Work out the finished part from the listing and answer in its coordinate system (mm). A direction names the side the tool comes from. Coordinates: 2 decimals unless noted, no trailing zeros. Loops run counter-clockwise (first coordinate to the right, second up) from the corner with the lowest first, then second, coordinate; pieces in that order, holes last. Notation, with made-up numbers: (13.25, 4) - (17.25, 4) arc R19 ccw to (17.25, 11) - close; hole circle Ø8 at (21.25, 62). An arc over 180 degrees is marked (long way). Write each question's results on one line, items separated by ' | '. Start each with the question number.
1. A cutting plane is placed at A-A on y = -6.25. Determine the outline of the cut face in (x, z).
2. Determine the mould class of faces 1 (the cylindrical face through (8.69, -5.26, 1.48)), 2 (the cylindrical face through (-6.31, -5.26, 1.48)), 3 (the flat face through (0, 9, 9)), 4 (the flat face through (-15.5, 0, 9)) for opening direction Y: released by +Y, released by -Y, zero draft, split by the parting line, or undercut.
3. Which of the six approach directions +Z, -Z, +X, -X, +Y, -Y give full straight-line access (tool end or side, diameter ignored) to faces 5 (the flat face through (15.5, 0, 9)), 6 (the flat face through (0, 2, 4.4)), 7 (the flat face through (0, 0, 12))?
4. A cutting plane is placed at D-D on z = 16.5. Determine the outline of the cut face in (x, y).
5. A cutting plane is placed at B-B on x = 7.5. Determine the outline of the cut face in (y, z).
6. Each of these flat-tipped pins is pushed along its axis until it touches: P1, Ø4.5, axis at x = -7, y = -5, coming from the +Z side; P2, Ø6, axis at x = -6, z = 14, coming from the -Y side. Where does it stop, or does it pass through?
7. A cutting plane is placed at C-C on y = 0.5. Determine the outline of the cut face in (x, z), then the cut area to 3 significant figures.
8. Find the intervals of material crossed by line 1 along X through (y, z) = (-4.25, 4.75); line 2 along Y through (x, z) = (7.5, 1.55); line 3 along Z through (x, y) = (2.5, 3), in increasing order. Write a range as [from, to].
from build123d import *

# Parameters (mm, degrees)
CROQUIS1_W              = 31
CROQUIS1_H              = 18
SALIENTE_EXTRUIR1_DEPTH = 19
CROQUIS3_W              = 25.1
CROQUIS3_H              = 9
CORTAR_EXTRUIR1_DEPTH   = 16
CROQUIS4_W              = 31
CROQUIS4_H              = 1.4
CORTAR_EXTRUIR2_DEPTH   = 15.1
CROQUIS5_R              = 1.5
CORTAR_EXTRUIR3_DEPTH   = 20


with BuildPart() as part:
    # Croquis1 → Saliente-Extruir1 (new body)
    with BuildSketch(Plane.XY):
        Rectangle(CROQUIS1_W, CROQUIS1_H)
    extrude(amount=SALIENTE_EXTRUIR1_DEPTH)

    # Croquis3 → Cortar-Extruir1 (cut)
    with BuildSketch(Plane.XY.offset(19)):
        with Locations((0, -4.5)):
            Rectangle(CROQUIS3_W, CROQUIS3_H)
    extrude(amount=-CORTAR_EXTRUIR1_DEPTH, mode=Mode.SUBTRACT)

    # Croquis4 → Cortar-Extruir2 (cut)
    with BuildSketch(Plane.XZ.offset(9)):
        with Locations((0, 3.7)):
            Rectangle(CROQUIS4_W, CROQUIS4_H)
    extrude(amount=-CORTAR_EXTRUIR2_DEPTH, mode=Mode.SUBTRACT)

    # Croquis5 → Cortar-Extruir3 (cut, through all)
    with BuildSketch(Plane(origin=(0, 0, 0), x_dir=(-1, 0, 0), z_dir=(0, 0, -1))):
        with Locations((-7.5, -4.35)):
            Circle(CROQUIS5_R)
        with Locations((7.5, -4.35)):
            Circle(CROQUIS5_R)
    extrude(amount=-CORTAR_EXTRUIR3_DEPTH, mode=Mode.SUBTRACT)


solid = part.part
Values:
1) outline: (-15.5, 0) - (15.5, 0) - (15.5, 3) - (-15.5, 3) - close; (-15.5, 4.4) - (-12.55, 4.4) - (-12.55, 19) - (-15.5, 19) - close; (12.55, 4.4) - (15.5, 4.4) - (15.5, 19) - (12.55, 19) - close
2) face 1: undercut | face 2: undercut | face 3: released by +Y | face 4: zero draft
3) face 5: +Z, -Z, +X, +Y, -Y | face 6: +X, -X, -Y | face 7: +Z, -Y
4) outline: (-15.5, -9) - (-12.55, -9) - (-12.55, 0) - (12.55, 0) - (12.55, -9) - (15.5, -9) - (15.5, 9) - (-15.5, 9) - close
5) outline: (-9, 0) - (-5.85, 0) - (-5.85, 3) - (-9, 3) - close; (-2.85, 0) - (9, 0) - (9, 19) - (0, 19) - (0, 4.4) - (6.1, 4.4) - (6.1, 3) - (-2.85, 3) - close
6) P1: z = 3 | P2: y = 0
7) outline: (-15.5, 0) - (15.5, 0) - (15.5, 3) - (-15.5, 3) - close; (-15.5, 4.4) - (15.5, 4.4) - (15.5, 19) - (-15.5, 19) - close | area: 546 mm^2
8) line 1: [-15.5, -12.55], [12.55, 15.5] | line 2: [-9, -5.85], [-2.85, 9] | line 3: [0, 3], [4.4, 19]
